from build123d import *

# Parameters (mm, degrees)
SKETCH1_R           = 5.08
SKETCH1_R_2         = 1.778
BOSS_EXTRUDE1_DEPTH = 10.16
BOSS_EXTRUDE3_DEPTH = 12.7
SKETCH3_W           = 7.874
SKETCH3_H           = 7.874
CUT_EXTRUDE1_DEPTH  = 6.35
FILLET1_R           = 2.54


with BuildPart() as part:
    # Sketch1 → Boss-Extrude1 (new body)
    with BuildSketch(Plane.XY):
        with BuildLine():
            Line((-6.35, 12.7), (-6.35, 10.998522628))
            ThreePointArc((-6.35, 10.998522628), (0, -12.7), (6.35, 10.998522628))
            Line((6.35, 10.998522628), (6.35, 12.7))
            Line((6.35, 12.7), (6.35, 114.3))
            Line((6.35, 114.3), (-6.35, 114.3))
            Line((-6.35, 114.3), (-6.35, 12.7))
        make_face()
        Circle(SKETCH1_R, mode=Mode.SUBTRACT)
        with Locations((0, 8.128)):
            Circle(SKETCH1_R_2, mode=Mode.SUBTRACT)
        with Locations((8.128, 0)):
            Circle(SKETCH1_R_2, mode=Mode.SUBTRACT)
        with Locations((0, -8.128)):
            Circle(SKETCH1_R_2, mode=Mode.SUBTRACT)
        with Locations((-8.128, 0)):
            Circle(SKETCH1_R_2, mode=Mode.SUBTRACT)
    extrude(amount=BOSS_EXTRUDE1_DEPTH)

    # Sketch2 → Boss-Extrude3 (add)
    with BuildSketch(Plane.ZY.offset(-6.35)):
        Polygon((0, 124.46), (10.16, 114.3), (0, 114.3), align=None)
    extrude(amount=BOSS_EXTRUDE3_DEPTH)

    # Sketch3 → Cut-Extrude1 (cut)
    with BuildSketch(Plane.XY.offset(10.16)):
        with Locations((0, 25.4)):
            Rectangle(SKETCH3_W, SKETCH3_H)
    extrude(amount=-CUT_EXTRUDE1_DEPTH, mode=Mode.SUBTRACT)

    # Fillet1
    fillet1_edges = [part.edges().sort_by_distance(p)[0] for p in [
        (6.35, 10.998522628, 5.08),
        (-6.35, 10.998522628, 5.08),
    ]]
    fillet(fillet1_edges, radius=FILLET1_R)


solid = part.part
Design review of the part built by this model. Coordinates are the model's own, in mm. A direction names the side the tool comes from. Give positions to 0.01 mm unless a question says otherwise; leave off trailing zeros. Write each loop counter-clockwise with the first axis right and the second up, starting at its lowest first coordinate (ties: lowest second). Pieces come first, ordered by that corner, then holes. Notation, with made-up numbers: M -25,58 L 28,58 A23 cw 28,68 Z; hole C -35,41.25 d11. An arc over 180 degrees is marked long. Answer as a JSON object with one key per item and string values. Group by question number.
1) We need section B-B (y = 0). Give the boundary of the cut face in (x, z).
2) We need section D-D (z = 5.25). Give the boundary of the cut face in (x, y).
3) For line 1 along Y through (x, z) = (-0.75, 9.5); line 2 along Y through (x, z) = (1, 7.5); line 3 along Y through (x, z) = (0.75, 3), list the stretches that pass through material, from the lowest coordinate up.
4) Tool access review of faces 1 (the face through (0, 52, 10.16)), 2 (the face through (6.35, 69, 5)), 3 (the face through (-6.486, -0.681, 5.009)), 4 (the face through (-6.35, 69, 5)), 5 (the face through (0, 29.337, 7)): name each direction out of +Z, -Z, +X, -X, +Y, -Y from which nothing blocks a thin tool from reaching the whole face with its end or side.
5) We need section C-C (x = -8.75). Give the boundary of the cut face in (y, z).
6) Clearance check with flat-ended pins moving along their axes: pin 1 Ø3 at (x, y) = (-8.128, 0) entering from +Z (3 decimals); pin 2 Ø1.5 at (x, z) = (-4.5, 9) entering from -Y; pin 3 Ø3 at (y, z) = (66, 5.5) entering from -X; pin 4 Ø5 at (x, z) = (0.5, 5.5) entering from +Y. State where each tip first meets the part, or that it passes through.
7) We need section A-A (x = 0). Give the boundary of the cut face in (y, z).
8) Mouldability with a two-part tool opening along X and no side actions: class faces 6 (the face through (-0.448, -12.692, 5.009)), 7 (the face through (0.09, 119.45, 5.01)), 8 (the face through (-3.937, 25, 7)), 9 (the face through (3.937, 25, 7)) as released by +X, released by -X, zero draft, split by the parting line, or undercut.
Answer key:
{
 "1": {"outline": "M -12.7,0 L -9.91,0 L -9.91,10.16 L -12.7,10.16 Z; M -6.35,0 L -5.08,0 L -5.08,10.16 L -6.35,10.16 Z; M 5.08,0 L 6.35,0 L 6.35,10.16 L 5.08,10.16 Z; M 9.91,0 L 12.7,0 L 12.7,10.16 L 9.91,10.16 Z"},
 "2": {"outline": "M -7.41,10.32 A12.7 ccw long 7.41,10.32 A2.54 cw 6.35,12.38 L 6.35,119.21 L -6.35,119.21 L -6.35,12.38 A2.54 cw Z; hole C -8.13,0 d3.56; hole C 0,0 d10.16; hole M -3.94,21.46 L 3.94,21.46 L 3.94,29.34 L -3.94,29.34 Z; hole C 0,-8.13 d3.56; hole C 0,8.13 d3.56; hole C 8.13,0 d3.56"},
 "3": {"line 1": "y = -12.68 to -9.74, -6.52 to -5.02, 5.02 to 6.52, 9.74 to 21.46, 29.34 to 114.96", "line 2": "y = -12.66 to -9.6, -6.66 to -4.98, 4.98 to 6.66, 9.6 to 21.46, 29.34 to 116.96", "line 3": "y = -12.68 to -9.74, -6.52 to -5.02, 5.02 to 6.52, 9.74 to 121.46"},
 "4": {"face 1": "+Z, +X, -X, +Y, -Y", "face 2": "+Z, -Z, +X, +Y", "face 3": "+Z, -Z", "face 4": "+Z, -Z, -X, +Y", "face 5": "+Z"},
 "5": {"outline": "M -9.2,0 L -1.67,0 L -1.67,10.16 L -9.2,10.16 Z; M 1.67,0 L 9.2,0 L 9.2,10.16 L 1.67,10.16 Z"},
 "6": {"pin 1": "passes through", "pin 2": "stops at y = -12.13", "pin 3": "stops at x = -6.35", "pin 4": "stops at y = 121.46"},
 "7": {"outline": "M -12.7,0 L -9.91,0 L -9.91,10.16 L -12.7,10.16 Z; M -6.35,0 L -5.08,0 L -5.08,10.16 L -6.35,10.16 Z; M 5.08,0 L 6.35,0 L 6.35,10.16 L 5.08,10.16 Z; M 9.91,0 L 124.46,0 L 114.3,10.16 L 29.34,10.16 L 29.34,3.81 L 21.46,3.81 L 21.46,10.16 L 9.91,10.16 Z"},
 "8": {"face 6": "split by the parting line", "face 7": "zero draft", "face 8": "undercut", "face 9": "undercut"}
}
